Verification items for this drawing (mm, ordinates from the low corner). A direction names the side the tool comes from. Coordinates: 2 decimals unless noted, no trailing zeros. Write each loop counter-clockwise with the first axis right and the second up, starting at its lowest first coordinate (ties: lowest second). Pieces come first, ordered by that corner, then holes. Notation, with made-up numbers: M -38.75,-40 L -6.75,-40 A16 cw -6.75,-24 Z; hole C 11.25,-26 d9. An arc over 180 degrees is marked long. Put each result on its own line as item: value. Start each with the question number.
1) Mould release check, pull along X, two halves, no side actions. Record for the marked faces 1, 2 and 3: released by +X, released by -X, zero draft, split by the parting line, or undercut.
2) Gauge pin test, flat ends, axial feed: pin 1 (4.5 mm diameter, centred on x = 16.5, y = 8.5, fed in from -Z); pin 2 (3 mm diameter, centred on x = 22.5, y = 4.5, fed in from +Z); pin 3 (12 mm diameter, centred on x = 26, z = 15.5, fed in from +Y); pin 4 (12 mm diameter, centred on x = 43, z = 6.5, fed in from -Y). Record the tip position at first contact, or that the pin passes through.
3) Cross-section at B-B on z = 14. Record the cut outline in (x, y).
4) Scan lines: line 1 along X through (y, z) = (13.5, 14); line 2 along Z through (x, y) = (43, 5.5); line 3 along X through (y, z) = (12, 1.5). Record each from-to range of solid material in increasing order.
5) Set-up check for the marked faces 4, 5, 6 and 7: record each of +Z, -Z, +X, -X, +Y, -Y from which the full face is reachable in a straight line by a thin tool's end or side.
6) Cross-section at A-A on x = 7.5. Record the cut outline in (y, z), plus the area to 3 significant figures.
7) Cross-section at D-D on y = 11.25. Record the cut outline in (x, z).
8) Cross-section at C-C on y = 3.25. Record the cut outline in (x, z).
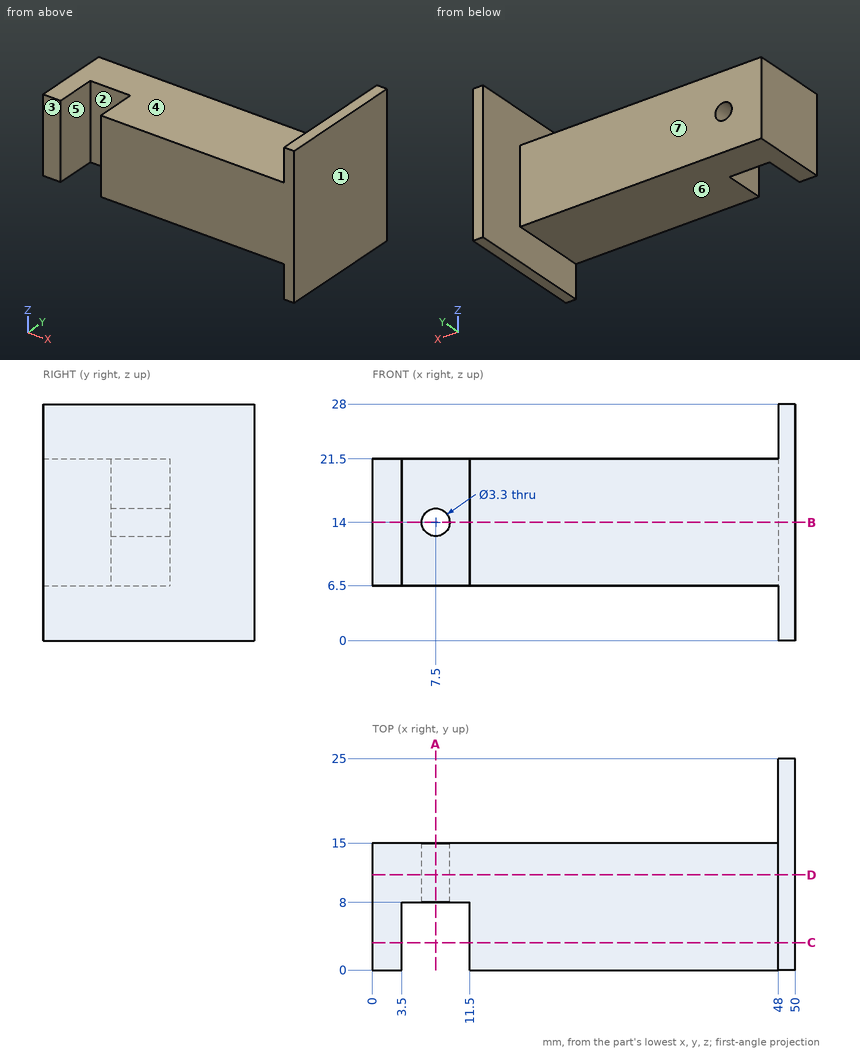
Answer key:
1. face 1: released by +X
1. face 2: undercut
1. face 3: zero draft
2. pin 1: stops at z = 6.5
2. pin 2: stops at z = 21.5
2. pin 3: stops at y = 15
2. pin 4: stops at y = 0
3. outline: M 0,0 L 3.5,0 L 3.5,8 L 5.85,8 L 5.85,15 L 0,15 Z; M 9.15,8 L 11.5,8 L 11.5,0 L 50,0 L 50,25 L 48,25 L 48,15 L 9.15,15 Z
4. line 1: x = 0 to 5.85, 9.15 to 50
4. line 2: z = 6.5 to 21.5
4. line 3: x = 48 to 50
5. face 4: +Z, -X, +Y, -Y
5. face 5: +Z, -Z, -Y
5. face 6: -Z, -X, +Y, -Y
5. face 7: +Z, -Z, -X, +Y
6. outline: M 8,6.5 L 15,6.5 L 15,12.35 L 8,12.35 Z; M 8,15.65 L 15,15.65 L 15,21.5 L 8,21.5 Z
6. area: 81.9 mm²
7. outline: M 0,6.5 L 48,6.5 L 48,0 L 50,0 L 50,28 L 48,28 L 48,21.5 L 0,21.5 Z; hole C 7.5,14 d3.3
8. outline: M 0,6.5 L 3.5,6.5 L 3.5,21.5 L 0,21.5 Z; M 11.5,6.5 L 48,6.5 L 48,0 L 50,0 L 50,28 L 48,28 L 48,21.5 L 11.5,21.5 Z
